```python
from build123d import *

# Parameters (mm, degrees)
SKETCH_1_R          = 3
EXTRUDE_1_DEPTH     = 5
SKETCH_2_R          = 2.5
CUT_EXTRUDE_1_DEPTH = 5
CUT_EXTRUDE_START   = -0.2
SKETCH_3_R          = 3
SKETCH_3_R_2        = 2.75
CUT_EXTRUDE_2_DEPTH = 0.2


with BuildPart() as part:
    # 草图1 → 凸台-拉伸1 (new body)
    with BuildSketch(Plane.XY):
        Circle(SKETCH_1_R)
    extrude(amount=EXTRUDE_1_DEPTH)

    # 草图2 → 切除-拉伸1 (cut)
    with BuildSketch(Plane(origin=(0, 0, 0), x_dir=(-1, 0, 0), z_dir=(0, 0, -1))):
        Circle(SKETCH_2_R)
    extrude(amount=-CUT_EXTRUDE_1_DEPTH, mode=Mode.SUBTRACT)

    # 草图3 → 切除-拉伸2 (cut)
    with BuildSketch(Plane.XY.offset(2.5).offset(CUT_EXTRUDE_START)):
        Circle(SKETCH_3_R)
        Circle(SKETCH_3_R_2, mode=Mode.SUBTRACT)
    extrude(amount=CUT_EXTRUDE_2_DEPTH, mode=Mode.SUBTRACT)


solid = part.part
```
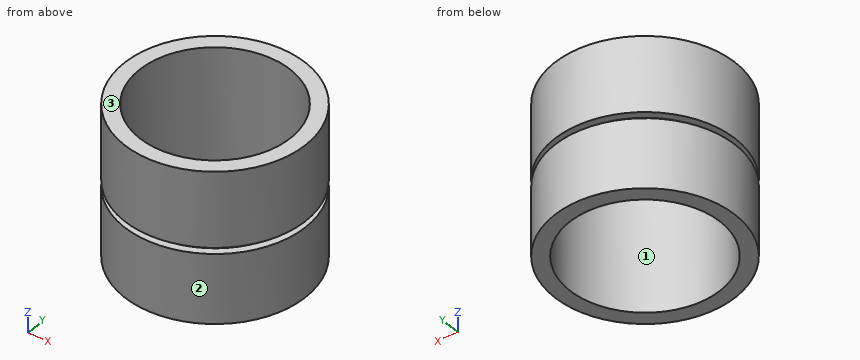
The listing builds one solid part. Answer for the finished solid, in the listing's coordinates (mm). Face numbers are marked on the shaded views. Coordinates: 2 decimals unless noted, no trailing zeros. Loops run counter-clockwise (first coordinate to the right, second up) from the corner with the lowest first, then second, coordinate; pieces in that order, holes last. Notation, with made-up numbers: (-0.5, -14.75) - (56.5, -14.75) arc R16 cw to (56.5, 11.25) - close; hole circle Ø8 at (-20.75, 36). An arc over 180 degrees is marked (long way). Write item = value, one per line.
1) Find the intervals of material crossed by line 1 along Z through (x, y) = (2.05, -2.05); line 2 along X through (y, z) = (0.1, 3.5), in increasing order.
Responses:
line_1 = 0 to 2.3, 2.5 to 5
line_2 = -3 to -2.5, 2.5 to 3
2) Section C-C (z = 1.8) is taken. Determine the outline of the cut face in (x, y).
Responses:
outline = circle Ø6 at (0, 0); hole circle Ø5 at (0, 0)
3) Determine the mould class of the marked faces 1, 2 and 3 for opening direction X: pulls with the +X half, pulls with the -X half, needs draft (parallel to the pull), parting line crosses it, or undercut.
Responses:
face_1 = undercut
face_2 = parting line crosses it
face_3 = needs draft
4) Section A-A (x = 0) is taken. Determine the outline of the cut face in (y, z).
Responses:
outline = (-3, 0) - (-2.5, 0) - (-2.5, 5) - (-3, 5) - (-3, 2.5) - (-2.75, 2.5) - (-2.75, 2.3) - (-3, 2.3) - close; (2.5, 0) - (3, 0) - (3, 2.3) - (2.75, 2.3) - (2.75, 2.5) - (3, 2.5) - (3, 5) - (2.5, 5) - close
5) Each of these flat-tipped pins is pushed along its axis until it touches: P1, Ø1.8, axis at x = 0.5, y = -0.5, coming from the +Z side; P2, Ø1, axis at y = -1.5, z = 3.5, coming from the +X side; P3, Ø2, axis at y = 1.5, z = 4, coming from the -X side. Where does it stop, or does it pass through?
Responses:
P1 = through
P2 = 2.83
P3 = -2.96
